Check sheet for the modelled part. Datum: model origin and axes. Units: mm. Face numbers are marked on the shaded views. Coordinates: 2 decimals unless noted, no trailing zeros. Loops run counter-clockwise (first coordinate to the right, second up) from the corner with the lowest first, then second, coordinate; pieces in that order, holes last. Notation, with made-up numbers: M 87,60 L 117,60 A10 cw 117,64 Z; hole C 86.25,50 d4. An arc over 180 degrees is marked long. Use CSV: the item, a comma, the result in double quotes. Start each with the question number.
(1) Section check B-B on y = 33. Record the cut outline in (x, z), and give its area (3 significant figures).
(2) Section check A-A on x = 85. Record the cut outline in (y, z), and give its area (3 significant figures).
(3) Section check C-C on x = 0. Record the cut outline in (y, z), and give its area (3 significant figures).
(4) Scan lines: line 1 (X direction, y = -25.5, z = 1); line 2 (Y direction, x = 0, z = 1.6); line 3 (X direction, y = -14.5, z = 4.8). Record each from-to range of solid material in increasing order.
(5) Draft check along Z on the marked faces 1 and 2. Enter one of: pulls with the +Z half, pulls with the -Z half, needs draft (parallel to the pull), parting line crosses it, or undercut.
(6) Section check D-D on y = 14. Record the cut outline in (x, z).
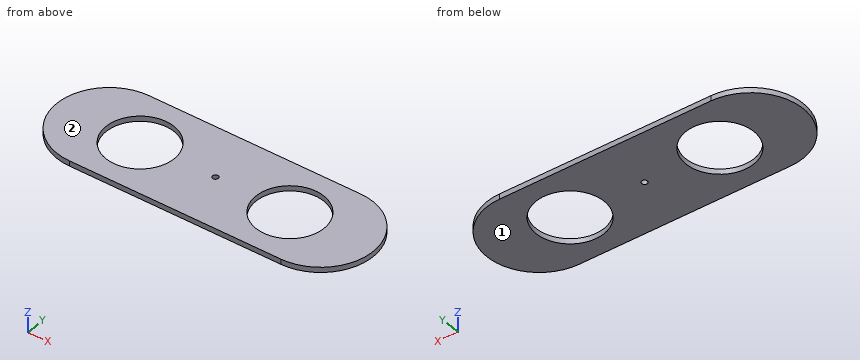
from build123d import *

# Parameters (mm, degrees)
BOSS_EXTRU_1_DEPTH      = 6
ENL_V_MAT_EXTRU_1_REACH = 191.832
ESQUISSE3_R             = 3.275
ENL_V_MAT_EXTRU_2_REACH = 191.832
ESQUISSE4_R             = 39


with BuildPart() as part:
    # Esquisse2 → Boss.-Extru.1 (new body)
    with BuildSketch(Plane.XY):
        with BuildLine():
            Line((120, -60), (-120, -60))
            ThreePointArc((-120, -60), (-180, 0), (-120, 60))
            Line((-120, 60), (120, 60))
            ThreePointArc((120, 60), (180, 0), (120, -60))
        make_face()
    extrude(amount=BOSS_EXTRU_1_DEPTH)

    # Esquisse3 → Enlèv. mat.-Extru.1 (cut, up to next)
    with BuildSketch(Plane.XY.offset(6), mode=Mode.PRIVATE) as enl_v_mat_extru_1_sk1:
        with Locations((0, 0.625)):
            Circle(ESQUISSE3_R)
    enl_v_mat_extru_1_tool1 = extrude(enl_v_mat_extru_1_sk1.sketch, amount=-ENL_V_MAT_EXTRU_1_REACH, mode=Mode.PRIVATE) & part.part
    add(enl_v_mat_extru_1_tool1.solids().sort_by_distance((0, 0.625, 6))[0], mode=Mode.SUBTRACT)

    # Esquisse4 → Enlèv. mat.-Extru.2 (cut, up to next)
    with BuildSketch(Plane.XY.offset(6), mode=Mode.PRIVATE) as enl_v_mat_extru_2_sk1:
        with Locations((-85, 0)):
            Circle(ESQUISSE4_R)
    enl_v_mat_extru_2_tool1 = extrude(enl_v_mat_extru_2_sk1.sketch, amount=-ENL_V_MAT_EXTRU_2_REACH, mode=Mode.PRIVATE) & part.part
    # Esquisse4 → Enlèv. mat.-Extru.2 (cut, up to next)
    with BuildSketch(Plane.XY.offset(6), mode=Mode.PRIVATE) as enl_v_mat_extru_2_sk2:
        with Locations((85, 0)):
            Circle(ESQUISSE4_R)
    enl_v_mat_extru_2_tool2 = extrude(enl_v_mat_extru_2_sk2.sketch, amount=-ENL_V_MAT_EXTRU_2_REACH, mode=Mode.PRIVATE) & part.part
    add(enl_v_mat_extru_2_tool1.solids().sort_by_distance((-85, 0, 6))[0], mode=Mode.SUBTRACT)
    add(enl_v_mat_extru_2_tool2.solids().sort_by_distance((85, 0, 6))[0], mode=Mode.SUBTRACT)


solid = part.part
Outcome:
1,outline,"M -170.11,0 L -105.78,0 L -105.78,6 L -170.11,6 Z; M -64.22,0 L 64.22,0 L 64.22,6 L -64.22,6 Z; M 105.78,0 L 170.11,0 L 170.11,6 L 105.78,6 Z"
1,area,"1,540 mm²"
2,outline,"M -60,0 L -39,0 L -39,6 L -60,6 Z; M 39,0 L 60,0 L 60,6 L 39,6 Z"
2,area,"252 mm²"
3,outline,"M -60,0 L -2.65,0 L -2.65,6 L -60,6 Z; M 3.9,0 L 60,0 L 60,6 L 3.9,6 Z"
3,area,"681 mm²"
4,line 1,"x = -174.31 to -114.51, -55.49 to 55.49, 114.51 to 174.31"
4,line 2,"y = -60 to -2.65, 3.9 to 60"
4,line 3,"x = -178.22 to -121.2, -48.8 to 48.8, 121.2 to 178.22"
5,face 1,"pulls with the -Z half"
5,face 2,"pulls with the +Z half"
6,outline,"M -178.34,0 L -121.4,0 L -121.4,6 L -178.34,6 Z; M -48.6,0 L 48.6,0 L 48.6,6 L -48.6,6 Z; M 121.4,0 L 178.34,0 L 178.34,6 L 121.4,6 Z"
